```python
from build123d import *

# Parameters (mm, degrees)
ESTRUSIONE_ESTRUSIONE1_DEPTH      = 5
ESTRUSIONE_ESTRUSIONE1_DEPTH_BACK = 5
ESTRUSIONE_ESTRUSIONE3_DEPTH      = 5
FORO_PER_VITE_M3_1_D              = 3.4
SCHIZZO26_W                       = 106.417777248
SCHIZZO26_H                       = 130
ESTRUSIONE_ESTRUSIONE5_DEPTH      = 2.5
NERVATURA2_REACH                  = 94.596
SCHIZZO29_WALL_W                  = 248.530633184
SCHIZZO29_WALL_H                  = 10
SMUSSO1_SIZE2                     = 6.868693549
SMUSSO1_SIZE                      = 2.5
RACCORDO1_R                       = 50
FORO_PER_VITE_M3_2_D              = 3.4


with BuildPart() as part:
    # Schizzo1 → Estrusione-Estrusione1 (new, two sides: drawn at the far end of the back side and taken through both)
    with BuildSketch(Plane.XY.offset(-ESTRUSIONE_ESTRUSIONE1_DEPTH_BACK)):
        Polygon((0, 0), (-100, 0), (-100, 38.897023427), (0, 2.5), align=None)
    extrude(amount=ESTRUSIONE_ESTRUSIONE1_DEPTH + ESTRUSIONE_ESTRUSIONE1_DEPTH_BACK)

    # Schizzo18 → Estrusione-Estrusione3 (add)
    with BuildSketch(Plane.XZ):
        with BuildLine():
            Line((-87.5, 5), (-72.5, 5))
            ThreePointArc((-72.5, 5), (-80, 12.5), (-87.5, 5))
        make_face()
    estrusione_estrusione3 = extrude(amount=-ESTRUSIONE_ESTRUSIONE3_DEPTH)

    # Foro per Vite M3-1 (through all)
    with Locations(Plane(origin=(-80, 5, 8.5), x_dir=(1, 0, 0), z_dir=(0, 1, 0))):
        with Locations((0, 0)):
            foro_per_vite_m3_1 = Hole(FORO_PER_VITE_M3_1_D / 2)

    # Specchia2: Estrusione-Estrusione3, Foro per Vite M3-1 across plane
    add(estrusione_estrusione3.mirror(Plane.XY))
    add(foro_per_vite_m3_1.mirror(Plane.XY), mode=Mode.SUBTRACT)

    # Schizzo26 → Estrusione-Estrusione5 (add)
    with BuildSketch(Plane(origin=(0.803484512, 2.207555554, 0), x_dir=(0.9396926207859082, -0.3420201433256694, 0), z_dir=(0.3420201433256694, 0.9396926207859083, 0))):
        with Locations((-54.063938982, 0)):
            Rectangle(SCHIZZO26_W, SCHIZZO26_H)
    extrude(amount=ESTRUSIONE_ESTRUSIONE5_DEPTH)

    # Schizzo29 wall → Nervatura2 (add, up to next)
    with BuildSketch(Plane(origin=(-41.11120737, 10.684369938, 35), x_dir=(0.071039265759, 0.195178778583, 0.978191528849), z_dir=(-0.334561206897, -0.919199361374, 0.207704917825)), mode=Mode.PRIVATE) as nervatura2_sk1:
        Rectangle(SCHIZZO29_WALL_W, SCHIZZO29_WALL_H)
    nervatura2_tool1 = extrude(nervatura2_sk1.sketch, amount=-NERVATURA2_REACH, mode=Mode.PRIVATE) - part.part
    nervatura2 = nervatura2_tool1.solids().sort_by_distance((-41.11120737, 10.684369938, 35))[0]
    add(nervatura2)

    # Specchia3: Nervatura2 across plane
    add(nervatura2.mirror(Plane.XY))

    # Smusso1
    smusso1_edges = [part.edges().sort_by_distance(p)[0] for p in [
        (0.855050358, 4.849231552, 0),
    ]]
    smusso1_side = [part.faces().sort_by_distance(p)[0] for p in [
        (0.837949351, 4.802246921, 0),
    ]]
    chamfer(smusso1_edges, length=SMUSSO1_SIZE - 0.0001, length2=SMUSSO1_SIZE2 - 0.0001, reference=smusso1_side[0])  # a hair under: the kernel refuses the full size

    # Raccordo1
    raccordo1_edges = [part.edges().sort_by_distance(p)[0] for p in [
        (-99.572474821, 40.071639203, -65),
        (-99.572474821, 40.071639203, 65),
    ]]
    fillet(raccordo1_edges, radius=RACCORDO1_R)

    # Foro per Vite M3-2 (through all)
    with Locations(Plane(origin=(1.65853487, 4.556787106, 0), x_dir=(0.9396926207859082, -0.3420201433256695, 0), z_dir=(0.3420201433256695, 0.9396926207859082, 0))):
        with Locations((-70.223743907, 57.5), (-70.223743907, -57.5), (-20.223743907, -57.5), (-20.223743907, 57.5)):
            Hole(FORO_PER_VITE_M3_2_D / 2)


solid = part.part
```
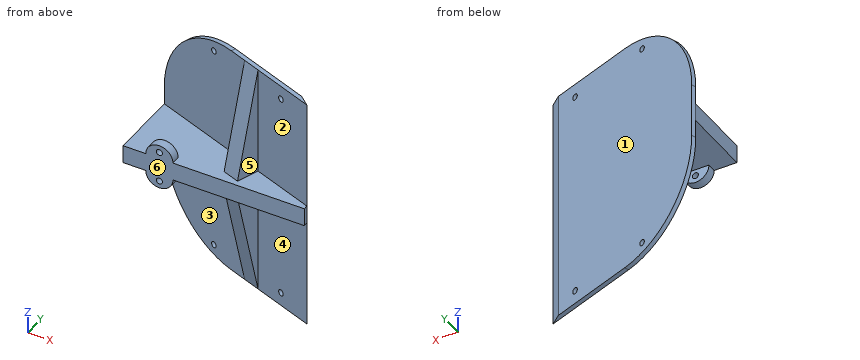
Check sheet for the modelled part. Datum: model origin and axes. Units: mm. Face numbers are marked on the shaded views. A direction names the side the tool comes from. Give positions to 0.01 mm unless a question says otherwise; leave off trailing zeros.
Item 1: Cross-section at A-A (z = 8.5). Count the separate pieces of the cut face and the enclosed holes in it, and give its area (3 significant figures).
Item 2: Access from +Z, -Z, +X, -X, +Y, -Y to the whole of each face (thin tool, end or side, straight path). Record for the marked faces 4, 5 and 6.
Item 3: Gauge pin test, flat ends, axial feed: pin 1 (2 mm diameter, centred on x = -80, z = -8.5, fed in from -Y); pin 2 (5 mm diameter, centred on x = -80.5, y = 31, fed in from -Z); pin 3 (3 mm diameter, centred on x = -72.5, z = 51.5, fed in from +Y). Record the tip position at first contact, or that the pin passes through.
Item 4: Draft check along X on the marked faces 1, 2 and 3. Enter one of: released by +X, released by -X, zero draft, split by the parting line, or undercut.
Item 5: Scan lines: L1, parallel to Z at x = -80, y = 1.25; L2, parallel to Z at x = -58.5, y = 5.5; L3, parallel to X at y = 1, z = -8. Record each from-to range of solid material in increasing order.
Report:
1. separate pieces: 3
1. enclosed holes: 0
1. area: 427 mm2
2. face 4: -Z, -Y
2. face 5: +Z, -Y
2. face 6: +Z, -Z, +X, -X, -Y
3. pin 1: stops at y = 31.25
3. pin 2: stops at z = -57.34
3. pin 3: stops at y = 32.09
4. face 1: released by +X
4. face 2: undercut
4. face 3: released by -X
5. L1: z = -12.5 to -10.2, -6.8 to 6.8, 10.2 to 12.5
5. L2: z = -5 to 5
5. L3: x = -86.87 to -81.62, -78.38 to -73.13
